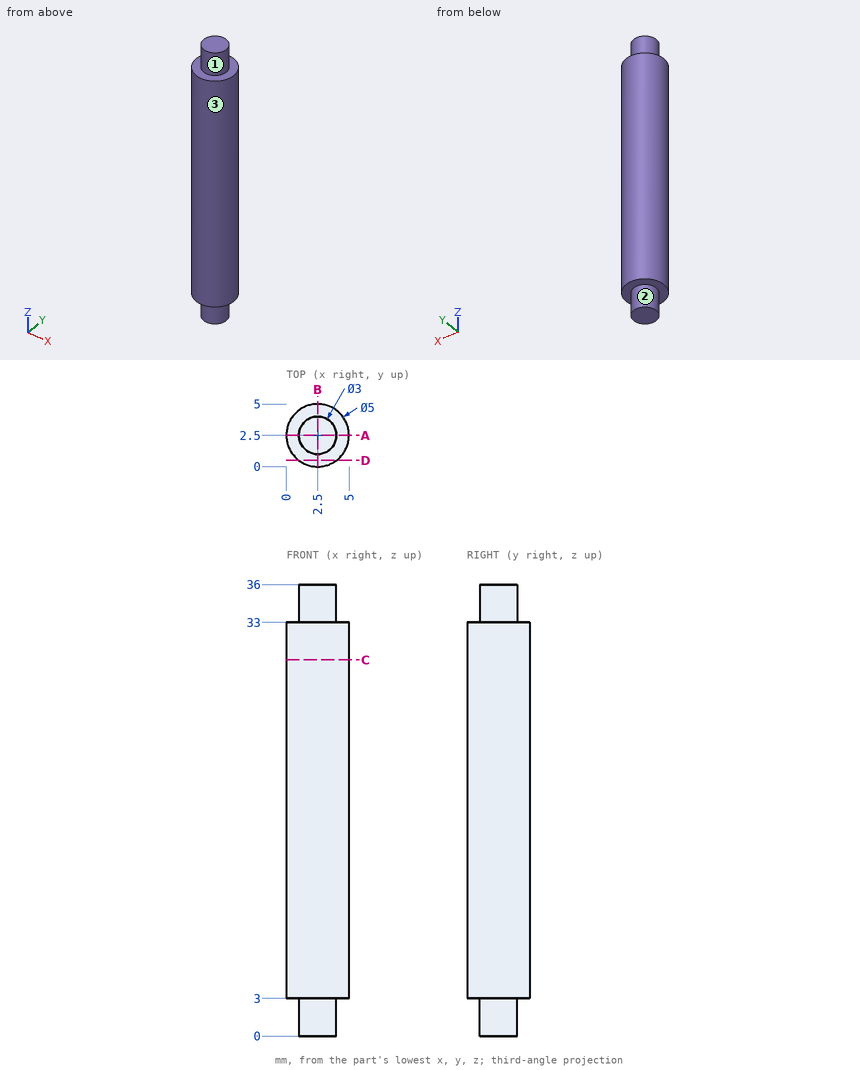
The drawing under review shows one solid part. Ordinate dimensions are in mm from its lowest x, y, z. A direction names the side the tool comes from. Coordinates: 2 decimals unless noted, no trailing zeros. Write each loop counter-clockwise with the first axis right and the second up, starting at its lowest first coordinate (ties: lowest second). Pieces come first, ordered by that corner, then holes. Notation, with made-up numbers: (-27.5, -6) -> (-12.5, -6) arc R13 ccw to (-12.5, 11) -> close; hole circle Ø4 at (60.25, 20.25). An arc over 180 degrees is marked (long way). Write each question's results on one line, items separated by ' | '. Start each with the question number.
1) Wall thickness on L1, parallel to Z at x = 3.35, y = 3.8; L2, parallel to X at y = 2.6, z = 14.5; L3, parallel to X at y = 4.5, z = 27.5: over which ranges is each line inside the solid? List them lowest first. Write a range as [from, to].
2) For the marked faces 1, 2 and 3, list the 3-axis set-ups (+Z, -Z, +X, -X, +Y, -Y) from which the entire face can be reached by the end or side of a thin tool; tool diameter is ignored.
3) Consider section C-C (z = 30). Write out the cut boundary in (x, y), plus the area to 3 significant figures.
4) Insertion check: pin 1 (3 mm diameter, centred on y = 4.5, z = 14, fed in from +X). The pin has a flat end and moves straight along its axis. Give the tip position at first contact, or say it passes through.
5) Consider section D-D (y = 0.5). Write out the cut boundary in (x, z).
6) Consider section A-A (y = 2.5). Write out the cut boundary in (x, z), plus the area to 3 significant figures.
Geometry says:
1) L1: [3, 33] | L2: [0, 5] | L3: [1, 4]
2) face 1: +Z | face 2: -Z | face 3: +Z, -Z
3) outline: circle Ø5 at (2.5, 2.5) | area: 19.6 mm^2
4) pin 1: x = 4.95
5) outline: (1, 3) -> (4, 3) -> (4, 33) -> (1, 33) -> close
6) outline: (0, 3) -> (1, 3) -> (1, 0) -> (4, 0) -> (4, 3) -> (5, 3) -> (5, 33) -> (4, 33) -> (4, 36) -> (1, 36) -> (1, 33) -> (0, 33) -> close | area: 168 mm^2
